Could you check a few things on this model? Use its own coordinates, in mm. Face numbers are marked on the shaded views. A direction names the side the tool comes from. Coordinates: 2 decimals unless noted, no trailing zeros. Loops run counter-clockwise (first coordinate to the right, second up) from the corner with the lowest first, then second, coordinate; pieces in that order, holes last. Notation, with made-up numbers: (-31, -12) -> (17, -12) arc R17 ccw to (17, -1) -> close; hole circle Ø10 at (69, -0.5). An arc over 180 degrees is marked (long way). One line per question, with ' | ' between items.
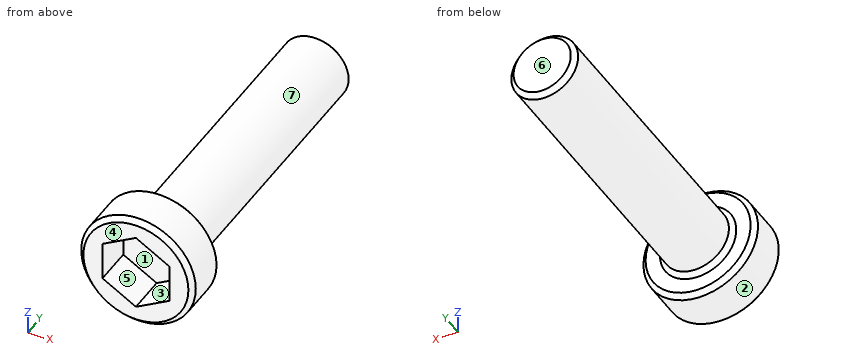
```python
from build123d import *

# Parameters (mm, degrees)
F0_R     = 3.5
F1_DEPTH = 30
F2_R     = 6
F3_DEPTH = 5
F4_SIZE  = 0.5
F6_DEPTH = 4


with BuildPart() as f1:
    # F0 (on Front) → F1 (new body)
    with BuildSketch(Plane.XZ):
        Circle(F0_R)
    extrude(amount=-F1_DEPTH)

    # F2 (on face) → F3 (join)
    with BuildSketch(Plane.XZ):
        Circle(F2_R)
    extrude(amount=F3_DEPTH)

    # F4
    f4_edges = [f1.edges().sort_by_distance(p)[0] for p in [
        (-6, -5, 0),
        (-6, 0, 0),
        (-3.5, 30, 0),
        (-3.5, 0, 0),
    ]]
    chamfer(f4_edges, length=F4_SIZE)

    # F5 (on face) → F6 (cut)
    with BuildSketch(Plane.XZ.offset(5)):
        Polygon((-3.5, 2.020726), (-3.5, -2.020726), (0, -4.041452), (3.5, -2.020726), (3.5, 2.020726), (0, 4.041452), align=None)
    extrude(amount=-F6_DEPTH, mode=Mode.SUBTRACT)


solid = f1.part
```
Q1. We'd pull the mould along X, two halves only. Please class the marked faces 1, 2, 3 and 4: released by +X, released by -X, zero draft, split by the parting line, or undercut.
Values follow:
face 1: undercut | face 2: split by the parting line | face 3: undercut | face 4: zero draft
Q2. For the marked faces 5, 6 and 7, which set-ups out of +Z, -Z, +X, -X, +Y, -Y let a thin tool reach every point of the face, with its end or its side?
Values follow:
face 5: -Y | face 6: +Z, -Z, +X, -X, +Y | face 7: +Y
Q3. Imagine slicing it at A-A on z = 0. Write out the boundary of the cut face in (x, y), plus the area to 4 significant figures.
Values follow:
outline: (-6, -4.5) -> (-5.5, -5) -> (-3.5, -5) -> (-3.5, -1) -> (3.5, -1) -> (3.5, -5) -> (5.5, -5) -> (6, -4.5) -> (6, -0.5) -> (5.5, 0) -> (4, 0) -> (3.5, 0.5) -> (3.5, 29.5) -> (3, 30) -> (-3, 30) -> (-3.5, 29.5) -> (-3.5, 0.5) -> (-4, 0) -> (-5.5, 0) -> (-6, -0.5) -> close | area: 241.5 mm2
Q4. Imagine slicing it at B-B on y = -2.5. Write out the boundary of the cut face in (x, z), plus the area to 3 significant figures.
Values follow:
outline: circle Ø12 at (0, 0); hole (-3.5, -2.02) -> (0, -4.04) -> (3.5, -2.02) -> (3.5, 2.02) -> (0, 4.04) -> (-3.5, 2.02) -> close | area: 70.7 mm2
Q5. For pin 1 (4 mm diameter, centred on x = -1.5, y = 23, fed in from +Z); pin 2 (6 mm diameter, centred on y = 11.5, z = 1.5, fed in from -X); pin 3 (3.5 mm diameter, centred on x = 1, z = -1, fed in from -Y), each with a flat end and sliding along its axis, tell me the tip position at first contact or that it passes through.
Values follow:
pin 1: stops at z = 3.5 | pin 2: stops at x = -3.5 | pin 3: stops at y = -1
Q6. Imagine slicing it at C-C on y = 24.5. Write out the boundary of the cut face in (x, z), plus the area to 3 significant figures.
Values follow:
outline: circle Ø7 at (0, 0) | area: 38.5 mm2
Q7. Please list where these lines run through material, in increasing order: L1, parallel to Y at x = 2.5, z = 4.25; L2, parallel to Z at x = 0.5, y = -2.5; L3, parallel to Y at x = 1, z = -2.5. Write a range as [from, to].
Values follow:
L1: y = [-5, 0] | L2: z = [-5.98, -3.75], [3.75, 5.98] | L3: y = [-1, 30]
